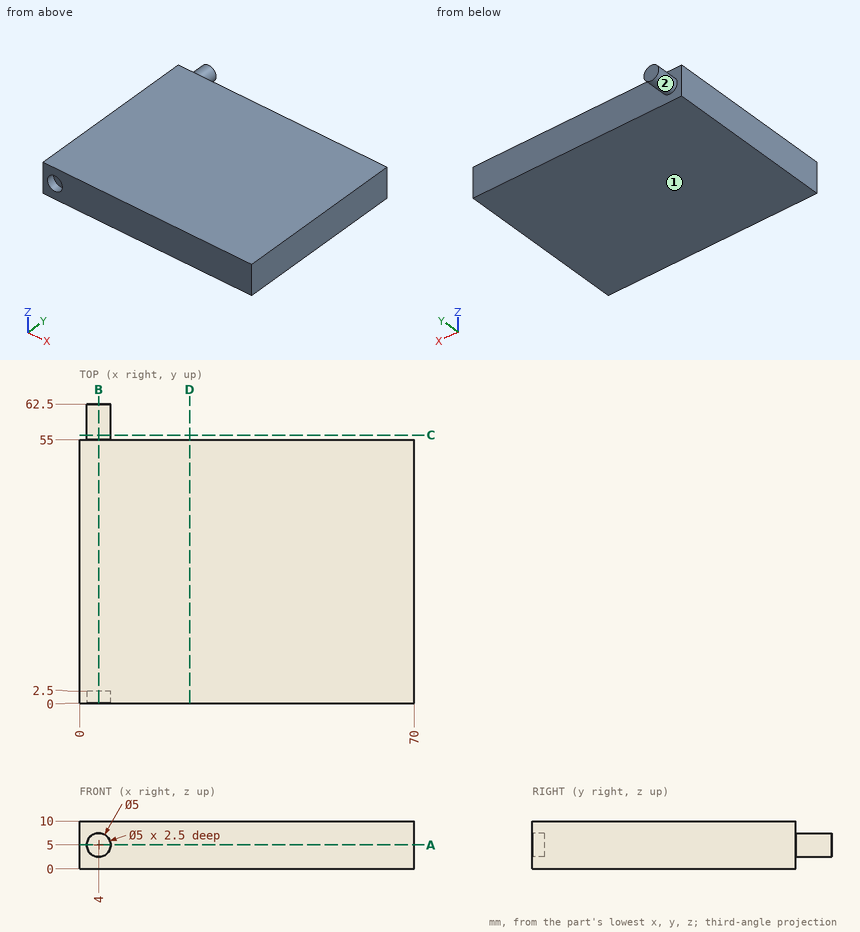
Check sheet for the drawn part. Datum: minimum x, y, z corner. Units: mm. A direction names the side the tool comes from. Give positions to 0.01 mm unless a question says otherwise; leave off trailing zeros. Loops run counter-clockwise (first coordinate to the right, second up) from the corner with the lowest first, then second, coordinate; pieces in that order, holes last.
1) Sectioned sample at C-C, the plane y = 56. Enter the section's corners in (x, z), then the cut area to 3 significant figures.
2) Sectioned sample at B-B, the plane x = 4. Enter the section's corners in (y, z), then the cut area to 3 significant figures.
3) Set-up check for the marked faces 1 and 2: record each of +Z, -Z, +X, -X, +Y, -Y from which the full face is reachable in a straight line by a thin tool's end or side.
4) Sectioned sample at A-A, the plane z = 5. Enter the section's corners in (x, y), then the cut area to 4 significant figures.
5) Depth check by flat-ended pin: pin 1 Ø4 at (x, z) = (23.5, 8.5) entering from +Y; pin 2 Ø3 at (x, z) = (4, 5) entering from -Y. Enter the tip coordinate at first touch or a pass-through.
6) Thickness scan on line 1 along Z through (x, y) = (4, 1.9); line 2 along X through (y, z) = (1.3, 5); line 3 along Y through (x, z) = (54, 9.75). Record the ranges inside material, lowest first.
7) Sectioned sample at D-D, the plane x = 23. Enter the section's corners in (y, z), then the cut area to 3 significant figures.
Answers:
1. outline: circle Ø5 at (4, 5)
1. area: 19.6 mm2
2. outline: (0, 0) - (55, 0) - (55, 2.5) - (62.5, 2.5) - (62.5, 7.5) - (55, 7.5) - (55, 10) - (0, 10) - (0, 7.5) - (2.5, 7.5) - (2.5, 2.5) - (0, 2.5) - close
2. area: 575 mm2
3. face 1: -Z, +X, -X, +Y, -Y
3. face 2: +Y
4. outline: (0, 0) - (1.5, 0) - (1.5, 2.5) - (6.5, 2.5) - (6.5, 0) - (70, 0) - (70, 55) - (6.5, 55) - (6.5, 62.5) - (1.5, 62.5) - (1.5, 55) - (0, 55) - close
4. area: 3,875 mm2
5. pin 1: stops at y = 55
5. pin 2: stops at y = 2.5
6. line 1: z = 0 to 2.5, 7.5 to 10
6. line 2: x = 0 to 1.5, 6.5 to 70
6. line 3: y = 0 to 55
7. outline: (0, 0) - (55, 0) - (55, 10) - (0, 10) - close
7. area: 550 mm2
